Source: CAD feature listing. Evaluate the final solid. Frame: model axes, mm. Face numbers are marked on the shaded views. A direction names the side the tool comes from. Round coordinates to 2 decimals unless told otherwise and drop trailing zeros. Order: outer loops, then holes, each group sorted by start corner. A loop starts at its lowest first (then second) coordinate and runs counter-clockwise, first axis right, second up.
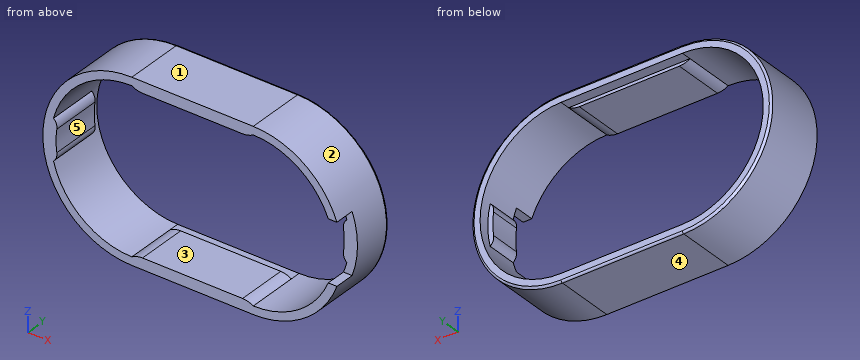
```python
from build123d import *

# Parameters (mm, degrees)
BOSS_EXTRUDE1_DEPTH = 30
SHELL1_T            = -4
SKETCH3_W           = 60
SKETCH3_H           = 1.5
BOSS_EXTRUDE2_DEPTH = 25
BOSS_EXTRUDE3_DEPTH = 25
FILLET2_R           = 10
BOSS_EXTRUDE5_DEPTH = 25
FILLET5_R           = 5
FILLET6_R           = 1
SKETCH9_W           = 17
SKETCH9_H           = 30
CUT_EXTRUDE1_DEPTH  = 10


with BuildPart() as part:
    # Sketch1 → Boss-Extrude1 (new body)
    with BuildSketch(Plane(origin=(0, 0, 0), x_dir=(1, 0, 0), z_dir=(0, 1, 0))):
        with BuildLine():
            Line((0, 0), (60, 0))
            ThreePointArc((60, 0), (104, 44), (60, 88))
            Line((60, 88), (0, 88))
            ThreePointArc((0, 88), (-44, 44), (0, 0))
        make_face()
    extrude(amount=BOSS_EXTRUDE1_DEPTH)

    # Shell1
    shell1_openings = [part.faces().sort_by_distance(p)[0] for p in [
        (30, 30, -44),
        (30, 0, -44),
    ]]
    offset(amount=SHELL1_T, openings=shell1_openings, kind=Kind.INTERSECTION)

    # Sketch3 → Boss-Extrude2 (add)
    with BuildSketch(Plane.XZ):
        with Locations((30, -4.75)):
            Rectangle(SKETCH3_W, SKETCH3_H)
    extrude(amount=-BOSS_EXTRUDE2_DEPTH)

    # Sketch5 → Boss-Extrude3 (add)
    with BuildSketch(Plane.XZ):
        Polygon((0, -84), (0, -82.5), (60.003782522, -82.5), (60, -84), align=None)
    extrude(amount=-BOSS_EXTRUDE3_DEPTH)

    # Fillet2
    # the kernel refuses this fillet: 10 mm, written as the material it takes off along each edge
    with BuildSketch(Plane(origin=(60, -13.169567191, -5.5), x_dir=(0, 0, 1), z_dir=(0, 1, 0)), Plane(origin=(0, -13.169567191, -82.5), x_dir=(0, 0, -1), z_dir=(0, 1, 0))) as fillet2_piece_1:
        with BuildLine():
            CenterArc((10, -5.267826876), FILLET2_R, 148.211669383, 31.788330617)
            Line((0, -5.267826876), (-0.2, -5.267826876))
            Line((-0.2, -5.267826876), (-0.2, 0))
            Line((-0.2, 0), (0, 0.2))
            ThreePointArc((0, 0.2), (0.75, 0.2), (1.33, 0.105356538))
            Line((1.33, 0.105356538), (1.5, 0))
        make_face()
    extrude(amount=51.339134382, mode=Mode.SUBTRACT)
    with BuildSketch(Plane(origin=(60.003782522, -13.179023495, -82.5), x_dir=(-1, 0, 0), z_dir=(0, 1, 0))) as fillet2_piece_2:
        with BuildLine():
            CenterArc((5.271609398, -10), FILLET2_R, 90, 31.788330617)
            Line((0.003782522, -1.5), (-0.101574016, -1.33))
            ThreePointArc((-0.101574016, -1.33), (-0.198108103, -0.750504335), (-0.199999364, -0.000504335))
            Line((-0.199999364, -0.000504335), (0, 0.2))
            Line((0, 0.2), (5.271609398, 0.2))
            Line((5.271609398, 0.2), (5.271609398, 0))
        make_face()
    extrude(amount=51.358046991, mode=Mode.SUBTRACT)
    with BuildSketch(Plane(origin=(0, -13.169567191, -5.5), x_dir=(1, 0, 0), z_dir=(0, 1, 0))) as fillet2_piece_3:
        with BuildLine():
            CenterArc((5.267826876, -10), FILLET2_R, 90, 31.788330617)
            Line((0, -1.5), (-0.105356538, -1.33))
            ThreePointArc((-0.105356538, -1.33), (-0.2, -0.75), (-0.2, 0))
            Line((-0.2, 0), (0, 0.2))
            Line((0, 0.2), (5.267826876, 0.2))
            Line((5.267826876, 0.2), (5.267826876, 0))
        make_face()
    extrude(amount=51.339134382, mode=Mode.SUBTRACT)

    # Sketch8 → Boss-Extrude5 (add)
    with BuildSketch(Plane.XZ):
        with BuildLine():
            Line((96.142080737, -34), (98.729833462, -34))
            ThreePointArc((98.729833462, -34), (100, -44), (98.729833462, -54))
            Line((98.729833462, -54), (96.142080737, -54))
            ThreePointArc((96.142080737, -54), (97.5, -44), (96.142080737, -34))
        make_face()
        with BuildLine():
            Line((-36.142080737, -54), (-38.729833462, -54))
            ThreePointArc((-38.729833462, -54), (-40, -44), (-38.729833462, -34))
            Line((-38.729833462, -34), (-36.142080737, -34))
            ThreePointArc((-36.142080737, -34), (-37.5, -44), (-36.142080737, -54))
        make_face()
    extrude(amount=-BOSS_EXTRUDE5_DEPTH)

    # Fillet5
    # the kernel refuses this fillet: 5 mm, written as the material it takes off along each edge
    with BuildSketch(Plane(origin=(96.142080737, -11.460527233, -34), x_dir=(1, 0, 0), z_dir=(0, 1, 0)), Plane(origin=(-36.142080737, -11.460527233, -54), x_dir=(-1, 0, 0), z_dir=(0, 1, 0))) as fillet5_piece_1:
        with BuildLine():
            CenterArc((5.895743435, 3.749292929), FILLET5_R, 171.542516957, 57.035612676)
            Line((0.950117062, 4.484670231), (0.851204534, 4.499377777))
            ThreePointArc((0.851204534, 4.499377777), (0.445822951, 2.248528932), (-0.096378882, 0.026666667))
            Line((-0.096378882, 0.026666667), (0, -0.1))
            ThreePointArc((0, -0.1), (1.293876363, -0.1), (2.521592911, -0.074985859))
            Line((2.521592911, -0.074985859), (2.587752725, 0))
        make_face()
    extrude(amount=47.921054465, mode=Mode.SUBTRACT)
    with BuildSketch(Plane(origin=(96.142080737, -11.460527233, -54), x_dir=(1, 0, 0), z_dir=(0, 1, 0)), Plane(origin=(-36.142080737, -11.460527233, -34), x_dir=(-1, 0, 0), z_dir=(0, 1, 0))) as fillet5_piece_2:
        with BuildLine():
            CenterArc((5.895743435, -3.749292929), FILLET5_R, 131.421870366, 57.035612676)
            Line((0.950117062, -4.484670231), (0.851204534, -4.499377777))
            ThreePointArc((0.851204534, -4.499377777), (0.445822951, -2.248528932), (-0.096378882, -0.026666667))
            Line((-0.096378882, -0.026666667), (0, 0.1))
            ThreePointArc((0, 0.1), (1.293876363, 0.1), (2.521592911, 0.074985859))
            Line((2.521592911, 0.074985859), (2.587752725, 0))
        make_face()
    extrude(amount=47.921054465, mode=Mode.SUBTRACT)

    # Fillet6
    fillet6_edges = [part.edges().sort_by_distance(p)[0] for p in [
        (104, 30, -44),
        (30, 30, -88),
        (-44, 30, -44),
        (30, 30, 0),
    ]]
    fillet(fillet6_edges, radius=FILLET6_R)

    # Sketch9 → Cut-Extrude1 (cut)
    with BuildSketch(Plane.XZ):
        with Locations((102.218118592, -44)):
            Rectangle(SKETCH9_W, SKETCH9_H)
    extrude(amount=-CUT_EXTRUDE1_DEPTH, mode=Mode.SUBTRACT)


solid = part.part
```
1. Section B-B on y = 20.75. Return loops of the section in (x, z).
2. Pull-direction query (X, two-part tool) for the marked faces 1, 2 and 3; classes: released by +X, released by -X, zero draft, split by the parting line, or undercut.
3. First-contact query: pin 1 (1.3 mm diameter, centred on x = 99.5, y = 7.5, fed in from +Z); pin 2 (1.5 mm diameter, centred on x = -5, y = 17.5, fed in from +Z); pin 3 (12 mm diameter, centred on x = -8, y = 6.5, fed in from -Z); pin 4 (1.2 mm diameter, centred on x = 34.5, z = -4.5, fed in from +Y). Flat tips, straight axial feed; report the tip coordinate or a pass-through.
4. Section A-A on z = -44. Return loops of the section in (x, y).
5. Access query for the marked faces 4 and 5. Directions: +Z, -Z, +X, -X, +Y, -Y. A direction counts if a zero-diameter tool reaches every point of the face in a straight line with its end or side. Return the directions, or none.
6. Section C-C on x = 47.5. Return loops of the section in (y, z).
7. Line query: line 1 along Z through (x, y) = (45, 5.25); line 2 along Z through (x, y) = (-1, 3.5); line 3 along X through (y, z) = (23, -28.5). Output: solid intervals per line, ascending.
Result:
1. outline: (0, -88) - (60, -88) arc R44 ccw to (60, 0) - (0, 0) arc R44 ccw to start; hole (-38.73, -54) arc R40 ccw to (0, -84) arc R10 cw to (5.27, -82.5) - (54.73, -82.5) arc R10 cw to (60, -84) arc R40 ccw to (98.73, -54) arc R5 cw to (97.09, -49.52) arc R37.5 ccw to (97.09, -38.48) arc R5 cw to (98.73, -34) arc R40 ccw to (60, -4) arc R10 cw to (54.73, -5.5) - (5.27, -5.5) arc R10 cw to (0, -4) arc R40 ccw to (-38.73, -34) arc R5 cw to (-37.09, -38.48) arc R37.5 ccw to (-37.09, -49.52) arc R5 cw to start
2. face 1: zero draft
2. face 2: released by +X
2. face 3: undercut
3. pin 1: stops at z = -23.34
3. pin 2: stops at z = -0.21
3. pin 3: stops at z = -87.95
3. pin 4: stops at y = 30
4. outline: (-44, 0) - (-37.5, 0) - (-37.5, 25) - (-40, 25) - (-40, 30) - (-43, 30) arc R1 ccw to (-44, 29) - close; (97.5, 10) - (104, 10) - (104, 29) arc R1 ccw to (103, 30) - (100, 30) - (100, 25) - (97.5, 25) - close
5. face 4: -Z, +X, -X, +Y, -Y
5. face 5: +Y, -Y
6. outline: (0, -88) - (29, -88) arc R1 ccw to (30, -87) - (30, -84) - (25, -84) - (25, -82.5) - (0, -82.5) - close; (0, -5.5) - (25, -5.5) - (25, -4) - (30, -4) - (30, -1) arc R1 ccw to (29, 0) - (0, 0) - close
7. line 1: z = -88 to -82.5, -5.5 to 0
7. line 2: z = -87.99 to -83.99, -4.01 to -0.01
7. line 3: x = -41.18 to -36.87, 96.87 to 101.18
